```python
from build123d import *

# Parameters (mm, degrees)
FILLET1_R = 1.25


with BuildPart() as part:
    # Sketch1 → Revolve1 (revolve)
    with BuildSketch(Plane.YZ, mode=Mode.PRIVATE) as revolve1_sk:
        with BuildLine():
            Line((0, 0), (0, 85.55))
            Line((0, 85.55), (3.18, 85.55))
            Line((3.18, 85.55), (3.18, 17.954698654))
            ThreePointArc((3.18, 17.954698654), (9.896609701, 5.315721242), (24.13, 3.81))
            Line((24.13, 3.81), (26.67, 1.27))
            Line((26.67, 1.27), (26.67, 0))
            Line((26.67, 0), (0, 0))
        make_face()
    revolve(revolve1_sk.sketch.rotate(Axis((0, 0, 0), (0, 0, 1)), 90), axis=Axis((0, 0, 0), (0, 0, 1)))

    # Fillet1
    fillet1_edges = [part.edges().sort_by_distance(p)[0] for p in [
        (3.18, 0, 85.55),
    ]]
    fillet(fillet1_edges, radius=FILLET1_R)


solid = part.part
```
Geometry check sheet. Reference: the model listing, model coordinates, mm. Round coordinates to 2 decimals unless told otherwise and drop trailing zeros. Loops run counter-clockwise (first coordinate to the right, second up) from the corner with the lowest first, then second, coordinate; pieces in that order, holes last. Notation, with made-up numbers: (84, 77.25) -> (93, 77.25) arc R22 ccw to (93, 99.25) -> close; hole circle Ø6 at (85.25, -12). An arc over 180 degrees is marked (long way). Use a Markdown table: item, result.
(1) Scan lines: probe 1 along Z at (x, y) = (-17, -8.5); probe 2 along Y at (x, z) = (2, 24.5); probe 3 along Z at (x, y) = (12, 10). Record each from-to range of solid material in increasing order.
Calculated:
| item | result |
|---|---|
| probe 1 | 0 to 2.72 |
| probe 2 | -2.47 to 2.47 |
| probe 3 | 0 to 2.97 |
(2) Sectioned sample at C-C (z = 79). Enter the section's corners in (x, y), then the cut area to 3 significant figures.
Calculated:
| item | result |
|---|---|
| outline | circle Ø6.36 at (0, 0) |
| area | 31.8 mm² |
(3) Mould release check, pull along Z, two halves, no side actions. Record for faces 1 (the cylindrical face through (2.524, 1.935, 50.663)), 2 (the flat face through (0, 0, 0)), 3 (the conical face through (-23.17, -7.3, 3.65)): released by +Z, released by -Z, zero draft, split by the parting line, or undercut.
Calculated:
| item | result |
|---|---|
| face 1 | zero draft |
| face 2 | released by -Z |
| face 3 | released by +Z |
(4) Sectioned sample at A-A (y = 0). Enter the section's corners in (x, z).
Calculated:
| item | result |
|---|---|
| outline | (-26.67, 0) -> (26.67, 0) -> (26.67, 1.27) -> (24.13, 3.81) arc R15.25 cw to (3.18, 17.95) -> (3.18, 84.3) arc R1.25 ccw to (1.93, 85.55) -> (-1.93, 85.55) arc R1.25 ccw to (-3.18, 84.3) -> (-3.18, 17.95) arc R15.25 cw to (-24.13, 3.81) -> (-26.67, 1.27) -> close |
(5) Go/stop test with flat-tipped pins: P1, Ø1.5, axis at x = -17, y = 17, coming from the +Z side; P2, Ø4, axis at x = 13, y = -14.5, coming from the +Z side; P3, Ø3, axis at y = 4, z = 32, coming from the -X side. Record where each tip stops, or that it passes through.
Calculated:
| item | result |
|---|---|
| P1 | z = 3.81 |
| P2 | z = 3.01 |
| P3 | x = -1.97 |
